Source: CAD feature listing. Evaluate the final solid. Frame: model axes, mm. Face numbers are marked on the shaded views. A direction names the side the tool comes from. Round coordinates to 2 decimals unless told otherwise and drop trailing zeros. Loops run counter-clockwise (first coordinate to the right, second up) from the corner with the lowest first, then second, coordinate; pieces in that order, holes last. Notation, with made-up numbers: (2, -18) -> (38, -18) arc R17 cw to (38, 0) -> close; hole circle Ø4 at (38, 39). An arc over 180 degrees is marked (long way). Return JSON: item names as keys, results as strings. Group by question number.
```python
from build123d import *

# Parameters (mm, degrees)
BOSS_EXTRUDE1_DEPTH = 11
SHELL1_T            = -4
FILLET1_R           = 7.5
BOSS_EXTRUDE2_START = 5
BOSS_EXTRUDE2_DEPTH = 5
SKETCH3_W           = 86
SKETCH3_H           = 55
CUT_EXTRUDE1_DEPTH  = 10
SKETCH4_R           = 12.5
SKETCH4_R_2         = 6.5
CUT_EXTRUDE2_DEPTH  = 10
FILLET2_R           = 2


with BuildPart() as part:
    # Sketch1 → Boss-Extrude1 (new body)
    with BuildSketch(Plane.XY):
        with BuildLine():
            Line((-32.761189707, -78.36284634), (-6.76388227, -109.345230875))
            ThreePointArc((-6.76388227, -109.345230875), (-4.18818591, -111.321632205), (-1.018548947, -112.024323803))
            Line((-1.018548947, -112.024323803), (131.986836181, -112.024323803))
            ThreePointArc((131.986836181, -112.024323803), (135.156473144, -111.321632205), (137.732169504, -109.345230875))
            Line((137.732169504, -109.345230875), (163.72947694, -78.36284634))
            ThreePointArc((163.72947694, -78.36284634), (165.031838273, -76.107090343), (165.484143617, -73.541939268))
            Line((165.484143617, -73.541939268), (165.484143617, -19.524323803))
            ThreePointArc((165.484143617, -19.524323803), (163.287444476, -14.221022944), (157.984143617, -12.024323803))
            Line((157.984143617, -12.024323803), (-27.015856383, -12.024323803))
            ThreePointArc((-27.015856383, -12.024323803), (-32.319157242, -14.221022944), (-34.515856383, -19.524323803))
            Line((-34.515856383, -19.524323803), (-34.515856383, -73.541939268))
            ThreePointArc((-34.515856383, -73.541939268), (-34.063551039, -76.107090343), (-32.761189707, -78.36284634))
        make_face()
    extrude(amount=BOSS_EXTRUDE1_DEPTH)

    # Shell1
    shell1_openings = [part.faces().sort_by_distance(p)[0] for p in [
        (65.484143617, -59.914594693, 0),
    ]]
    offset(amount=SHELL1_T, openings=shell1_openings, kind=Kind.INTERSECTION)

    # Fillet1
    fillet1_edges = [part.edges().sort_by_distance(p)[0] for p in [
        (135.156473144, -111.321632205, 11),
        (150.730823222, -93.854038608, 11),
        (165.031838273, -76.107090343, 11),
        (165.484143617, -46.533131535, 11),
        (163.287444476, -14.221022944, 11),
        (65.484143617, -12.024323803, 11),
        (-32.319157242, -14.221022944, 11),
        (-34.515856383, -46.533131535, 11),
        (-34.063551039, -76.107090343, 11),
        (-19.762535988, -93.854038608, 11),
        (-4.18818591, -111.321632205, 11),
        (65.484143617, -112.024323803, 11),
    ]]
    fillet(fillet1_edges, radius=FILLET1_R)

    # Sketch2 → Boss-Extrude2 (add)
    with BuildSketch(Plane(origin=(0, 0, 0), x_dir=(-1, 0, 0), z_dir=(0, 0, -1)).offset(BOSS_EXTRUDE2_START)):
        with BuildLine():
            Line((5.231793384, -108.059655656), (31.22910082, -77.077271121))
            ThreePointArc((31.22910082, -77.077271121), (32.184165797, -75.423050056), (32.515856383, -73.541939268))
            Line((32.515856383, -73.541939268), (32.515856383, -19.524323803))
            ThreePointArc((32.515856383, -19.524323803), (30.90494368, -15.635236506), (27.015856383, -14.024323803))
            Line((27.015856383, -14.024323803), (-157.984143617, -14.024323803))
            ThreePointArc((-157.984143617, -14.024323803), (-161.873230913, -15.635236506), (-163.484143617, -19.524323803))
            Line((-163.484143617, -19.524323803), (-163.484143617, -73.541939268))
            ThreePointArc((-163.484143617, -73.541939268), (-163.152453031, -75.423050056), (-162.197388054, -77.077271121))
            Line((-162.197388054, -77.077271121), (-136.200080618, -108.059655656))
            ThreePointArc((-136.200080618, -108.059655656), (-134.31123662, -109.509016631), (-131.986836181, -110.024323803))
            Line((-131.986836181, -110.024323803), (1.018548947, -110.024323803))
            ThreePointArc((1.018548947, -110.024323803), (3.342949387, -109.509016631), (5.231793384, -108.059655656))
        make_face()
        with BuildLine():
            Line((3.699704498, -106.774080437), (29.697011934, -75.791695902))
            ThreePointArc((29.697011934, -75.791695902), (30.304780556, -74.739009769), (30.515856383, -73.541939268))
            Line((30.515856383, -73.541939268), (30.515856383, -19.524323803))
            ThreePointArc((30.515856383, -19.524323803), (29.490730117, -17.049450068), (27.015856383, -16.024323803))
            Line((27.015856383, -16.024323803), (-157.984143617, -16.024323803))
            ThreePointArc((-157.984143617, -16.024323803), (-160.459017351, -17.049450068), (-161.484143617, -19.524323803))
            Line((-161.484143617, -19.524323803), (-161.484143617, -73.541939268))
            ThreePointArc((-161.484143617, -73.541939268), (-161.27306779, -74.739009769), (-160.665299168, -75.791695902))
            Line((-160.665299168, -75.791695902), (-134.667991732, -106.774080437))
            ThreePointArc((-134.667991732, -106.774080437), (-133.466000097, -107.696401057), (-131.986836181, -108.024323803))
            Line((-131.986836181, -108.024323803), (1.018548947, -108.024323803))
            ThreePointArc((1.018548947, -108.024323803), (2.497712863, -107.696401057), (3.699704498, -106.774080437))
        make_face(mode=Mode.SUBTRACT)
    extrude(amount=-BOSS_EXTRUDE2_DEPTH)

    # Sketch3 → Cut-Extrude1 (cut)
    with BuildSketch(Plane.XY.offset(11)):
        with Locations((65.734143617, -60.524323803)):
            Rectangle(SKETCH3_W, SKETCH3_H)
    extrude(amount=-CUT_EXTRUDE1_DEPTH, mode=Mode.SUBTRACT)

    # Sketch4 → Cut-Extrude2 (cut)
    with BuildSketch(Plane.XY.offset(11)):
        with Locations((-3.765856383, -41.224323803)):
            Circle(SKETCH4_R)
        with Locations((-8.183616573, -70.961609401)):
            Circle(SKETCH4_R_2)
        with Locations((4.218548656, -86.65193437)):
            Circle(SKETCH4_R_2)
        with Locations((127.249738577, -86.65193437)):
            Circle(SKETCH4_R_2)
        with Locations((139.651903807, -70.961609401)):
            Circle(SKETCH4_R_2)
        with Locations((135.234143617, -41.224323803)):
            Circle(SKETCH4_R)
    extrude(amount=-CUT_EXTRUDE2_DEPTH, mode=Mode.SUBTRACT)

    # Fillet2
    fillet2_edges = [part.edges().sort_by_distance(p)[0] for p in [
        (122.734143617, -41.224323803, 7),
        (122.734143617, -41.224323803, 11),
        (-16.265856383, -41.224323803, 7),
        (-16.265856383, -41.224323803, 11),
    ]]
    fillet(fillet2_edges, radius=FILLET2_R - 0.0001)  # a hair under: the kernel refuses the full size


solid = part.part
```
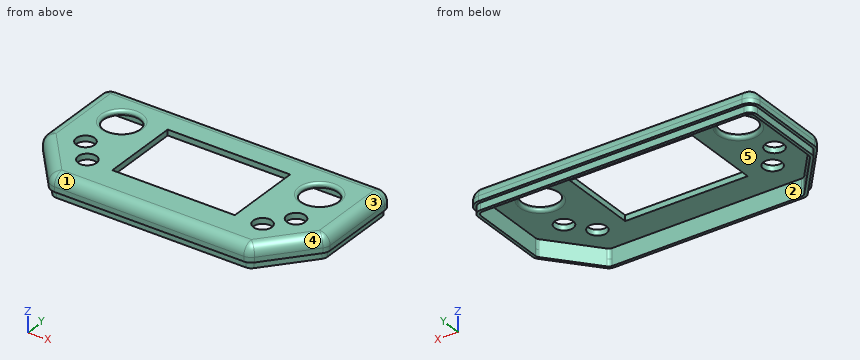
(1) Cut plane A-A (x = 53). Return loops of the section in (y, z), and give its area (3 significant figures).
(2) Set-up query: the marked faces 1 and 2. Return all of +Z, -Z, +X, -X, +Y, -Y with unobstructed straight access to the full face (end or side cutting, diameter ignored); none if empty.
(3) Mould query, pull axis Y, two halves, no side actions, for the marked faces 3, 4 and 5. Classes: released by +Y, released by -Y, zero draft, split by the parting line, or undercut.
(4) Ray query, line 1 (Y direction, x = 79.5, z = -1.25); line 2 (Y direction, x = 103, z = 1.75); line 3 (X direction, y = -33, z = -4.5). Return the intervals inside material, ascending.
(5) Cut plane C-C (y = -37). Count the separate pieces of the cut face and the enclosed holes in it, and give its area (3 significant figures).
(6) Cut plane B-B (x = 114). Return loops of the section in (y, z), and give its area (3 significant figures).
(7) Pin query (flat end, axial travel): pin 1 (1.5 mm diameter, centred on y = -37.5, z = -2.5, fed in from +X); pin 2 (8 mm diameter, centred on x = 134.5, z = 8, fed in from -Y) (3 decimals); pin 3 (4.5 mm diameter, centred on x = 59, z = 9, fed in from +Y). Return the tip coordinate at first contact, or that it passes through.
Answers follow:
{
 "1": {"outline": "(-112.02, 0) -> (-110.02, 0) -> (-110.02, -5) -> (-108.02, -5) -> (-108.02, 7) -> (-88.02, 7) -> (-88.02, 11) -> (-104.52, 11) arc R7.5 ccw to (-112.02, 3.5) -> close; (-33.02, 7) -> (-16.02, 7) -> (-16.02, -5) -> (-14.02, -5) -> (-14.02, 0) -> (-12.02, 0) -> (-12.02, 3.5) arc R7.5 ccw to (-19.52, 11) -> (-33.02, 11) -> close", "area": "232 mm^2"},
 "2": {"face 1": "+Z, +X, -X, -Y", "face 2": "-Z"},
 "3": {"face 3": "zero draft", "face 4": "released by -Y", "face 5": "undercut"},
 "4": {"line 1": "-110.02 to -108.02, -16.02 to -14.02", "line 2": "-112.02 to -108.02, -16.02 to -12.02", "line 3": "-32.52 to -30.52, 161.48 to 163.48"},
 "5": {"separate pieces": "4", "enclosed holes": "0", "area": "312 mm^2"},
 "6": {"outline": "(-112.02, 0) -> (-110.02, 0) -> (-110.02, -5) -> (-108.02, -5) -> (-108.02, 7) -> (-16.02, 7) -> (-16.02, -5) -> (-14.02, -5) -> (-14.02, 0) -> (-12.02, 0) -> (-12.02, 3.5) arc R7.5 ccw to (-19.52, 11) -> (-104.52, 11) arc R7.5 ccw to (-112.02, 3.5) -> close", "area": "452 mm^2"},
 "7": {"pin 1": "x = 163.48", "pin 2": "y = -111.935", "pin 3": "y = -12.77"}
}
